Autodesk Inventor part; units mm, degrees
ref_plane "YZ Plane" through (0, 0, 0) normal (1, 0, 0) x (0, 1, 0)
ref_plane "XZ Plane" through (0, 0, 0) normal (0, 1, 0) x (-1, 0, 0)
ref_plane "XY Plane" through (0, 0, 0) normal (0, 0, 1) x (1, 0, 0)
sketch "Sketch1" plane through (0, 0, 0) normal (0, 0, 1) x (1, 0, 0)
  circle A0 centre (0, 0) radius 228.5
  arc A1 (-325, 0) -> (325, 0) centre (0, 0) ccw
  line L0 (325, 0) -> (325, 1000)
  line L1 (325, 0) -> (1325, 0) construction
  line L2 (-267.2125, -184.9932) -> (732.7875, -184.9932) construction
  line L3 (-325, 0) -> (-325, 1000)
  line L4 (-325, 0) -> (675, 0) construction
  line L5 (-225, 1000) -> (225, 1000)
  line L6 (0, 1000) -> (-100, 1000)
  line L7 (-100, 1000) -> (-100, 1500)
  line L8 (0, 1000) -> (100, 1000)
  line L9 (100, 1000) -> (100, 1500)
  arc A2 (325, 1000) -> (325, 1528.4091) centre (-99.4949, 1264.2046) ccw
  arc A3 (225, 1000) -> (225, 1526.7827) centre (-200, 1263.3913) ccw
  arc A4 (-316.0183, 1540.7518) -> (-325, 1000) centre (100, 1263.3913) ccw
  arc A5 (-216.0183, 1540.7518) -> (-225, 1000) centre (200, 1263.3913) ccw
  line L10 (-216.0183, 1540.7518) -> (-166.9198, 1640.7518)
  line L11 (-166.9198, 1640.7518) -> (-316.0183, 1540.7518)
  line L12 (225, 1526.7827) -> (173.5917, 1612.5567)
  line L13 (173.5917, 1612.5567) -> (325, 1528.4091)
  line L14 (100, 1500) -> (1.2499, 1750)
  line L15 (1.2499, 1750) -> (-100, 1500)
  point P0 (100, 1250)
  dimension "d0" = 457
  dimension "d1" = 650
  dimension "d2" = 1000
  dimension "d3" = 90
  dimension "d6" = 1000
  dimension "d7" = 90
  dimension "d8" = 100
  dimension "d9" = 500
  dimension "d10" = 100
  dimension "d11" = 500
  dimension "d12" = 500
  dimension "d13" = 200
  dimension "d14" = 500
  dimension "d15" = 300
  dimension "d16" = 100
  dimension "d17" = 500
  dimension "d18" = 500
  dimension "d19" = 100
  dimension "d20" = 200
  dimension "d22" = 100
  dimension "d23" = 100
  dimension "d25" = 300
  dimension "d26" = 100
  dimension "d27" = 30
  dimension "d28" = 30
  dimension "d29" = 100
  dimension "d30" = 250
  dimension "d31" = 43.602
extrude "Extrusion1" add sketch "Sketch1" along normal blind 200
properties part number "The Gripper. (New)"
Geometry: final body of the model. Coordinates: model frame, mm. A direction names the side the tool comes from. Coordinates: 2 decimals unless noted, no trailing zeros. Loops run counter-clockwise (first coordinate to the right, second up) from the corner with the lowest first, then second, coordinate; pieces in that order, holes last. Notation, with made-up numbers: M -11.5,70 L 11.5,70 A27 ccw 11.5,106 Z; hole C -34.75,-5 d3. An arc over 180 degrees is marked long. Put each result on its own line as item: value.
(1) Draft query along X for faces 1 (the face through (-399.98, 1267.7, 98.6)), 2 (the face through (400.49, 1268.1, 98.6)), 3 (the face through (-5, 727, 200)), 4 (the face through (51.316, 1623.25, 98.6)). Return one class per face: pulls with the +X half, pulls with the -X half, needs draft (parallel to the pull), parting line crosses it, or undercut.
Answer sheet:
face 1: pulls with the -X half
face 2: pulls with the +X half
face 3: needs draft
face 4: undercut
(2) Cut plane B-B on z = 68. Return the cut outline in (x, y).
Answer sheet:
outline: M -325,0 A325 ccw 325,0 L 325,1000 A500 ccw 325,1528.41 L 173.59,1612.56 L 225,1526.78 A500 cw 225,1000 L 100,1000 L 100,1500 L 1.25,1750 L -100,1500 L -100,1000 L -225,1000 A500 cw -216.02,1540.75 L -166.92,1640.75 L -316.02,1540.75 A500 ccw -325,1000 Z; hole C 0,0 d457
(3) Cut plane D-D on x = 150.5. Return the cut outline in (y, z), then the cut area to 3 significant figures.
Answer sheet:
outline: M -288.05,0 L -171.94,0 L -171.94,200 L -288.05,200 Z; M 171.94,0 L 1000,0 L 1000,200 L 171.94,200 Z
area: 189,000 mm^2
(4) Cut plane A-A on y = 1306.5. Return the cut outline in (x, z), then the cut area to 3 significant figures.
Answer sheet:
outline: M -398.14,0 L -298.14,0 L -298.14,200 L -398.14,200 Z; M -100,0 L 100,0 L 100,200 L -100,200 Z; M 298.14,0 L 398.71,0 L 398.71,200 L 298.14,200 Z
area: 80,100 mm^2
(5) Cut plane C-C on y = 61.5. Return the cut outline in (x, z), then the cut area to 3 significant figures.
Answer sheet:
outline: M -325,0 L -220.07,0 L -220.07,200 L -325,200 Z; M 220.07,0 L 325,0 L 325,200 L 220.07,200 Z
area: 42,000 mm^2
(6) Material intervals for probe 1 along X at (y, z) = (1264, 54.5); probe 2 along X at (y, z) = (1598, 10.5); probe 3 along Y at (x, z) = (-115.5, 116), sorted ascending.
Answer sheet:
probe 1: x = -400 to -300, -100 to 100, 300 to 400.51
probe 2: x = -230.66 to -187.91, -60.31 to 61.29, 182.32 to 199.78
probe 3: y = -303.78 to -197.16, 197.16 to 1000
(7) Access query for faces 5 (the face through (-299.98, 1267.7, 98.6)), 6 (the face through (-100, 1246, 99)), 7 (the face through (325, 493, 99)). Directions: +Z, -Z, +X, -X, +Y, -Y. A direction counts if a zero-diameter tool reaches every point of the face in a straight line with its end or side. Return the directions, or none.
Answer sheet:
face 5: +Z, -Z
face 6: +Z, -Z, +Y
face 7: +Z, -Z, +X, -Y
(8) First-contact query: pin 1 (1 mm diameter, centred on y = 552, z = 68, fed in from -X); pin 2 (6 mm diameter, centred on x = -225.5, z = 127, fed in from -Y); pin 3 (1 mm diameter, centred on y = 704, z = 177, fed in from +X). Flat tips, straight axial feed; report the tip coordinate or a pass-through.
Answer sheet:
pin 1: stops at x = -325
pin 2: stops at y = -236.89
pin 3: stops at x = 325
